Autodesk Inventor part; units mm, degrees
ref_plane "YZ Plane" through (0, 0, 0) normal (1, 0, 0) x (0, 1, 0)
ref_plane "XZ Plane" through (0, 0, 0) normal (0, 1, 0) x (-1, 0, 0)
ref_plane "XY Plane" through (0, 0, 0) normal (0, 0, 1) x (1, 0, 0)
sketch "Sketch1" plane through (0, 0, 0) normal (0, 1, 0) x (-1, 0, 0)
  line L0 (46, 0) -> (-35, 0) construction
  line L1 (0, 54) -> (0, -60) construction
  line L2 (10, 20) -> (-10, 20)
  line L3 (-10, 20) -> (-10, -20)
  line L4 (-10, -20) -> (10, -20)
  line L5 (10, -20) -> (10, 20)
  line L6 (17, -28) -> (17, 28)
  line L7 (17, 28) -> (-13, 28)
  line L8 (-13, 28) -> (-13, -9.5)
  line L9 (-13, -9.5) -> (-36.5, -9.5)
  line L10 (-36.5, -9.5) -> (-36.5, -28)
  line L11 (-36.5, -28) -> (17, -28)
  line L12 (-29.5, -20) -> (-29.5, -17.5)
  line L13 (-10.5, -17.5) -> (-10.5, -20)
  circle A0 centre (5, 24.25) radius 0.5
  circle A1 centre (-5, 24.25) radius 0.5
  line L14 (14.6784, 24.25) -> (-18, 24.25) construction
  circle A2 centre (5, -24.25) radius 0.5
  circle A3 centre (-5, -24.25) radius 0.5
  circle A4 centre (13.5, -18.75) radius 1.5
  circle A5 centre (13.5, 18.75) radius 1.5
  circle A6 centre (-33, -18.75) radius 1.5
  line L15 (-20, 4) -> (-20, -26.5) construction
  line L16 (-10.5, -20) -> (-19.5, -20)
  line L17 (-19.5, -20) -> (-19.5, -22)
  line L18 (-19.5, -22) -> (-20.5, -22)
  line L19 (-20.5, -22) -> (-20.5, -20)
  line L20 (-20.5, -20) -> (-29.5, -20)
  line L21 (-10.5, -17.5) -> (-29.5, -17.5)
  point P0 (0, 0)
  point P1 (-20.5, -17.5)
  dimension "d0" = 40
  dimension "d1" = 20
  dimension "d2" = 7
  dimension "d3" = 8
  dimension "d4" = 8
  dimension "d5" = 3
  dimension "d6" = 20
  dimension "d7" = 10
  dimension "d8" = 19
  dimension "d9" = 2.5
  dimension "d10" = 0.5
  dimension "d11" = 1
  dimension "d12" = 1
  dimension "d13" = 5
  dimension "d14" = 5
  dimension "d15" = 4.25
  dimension "d16" = 3
  dimension "d17" = 9.25
  dimension "d19" = 18.5
  dimension "d20" = 7
  dimension "d21" = 3
  dimension "d23" = 9.25
  dimension "d29" = 3.5
  dimension "d30" = 3.5
  dimension "d31" = 2
  dimension "d32" = 1
extrude "Extrusion1" add sketch "Sketch1" along normal blind 3
fillet "Fillet1" radius 1 6 edges at (-17, 1.5, 28) (13, 1.5, 28) (13, 1.5, -9.5) (36.5, 1.5, -9.5) (36.5, 1.5, -28) (-17, 1.5, -28)
properties part number "BracketCoxa"
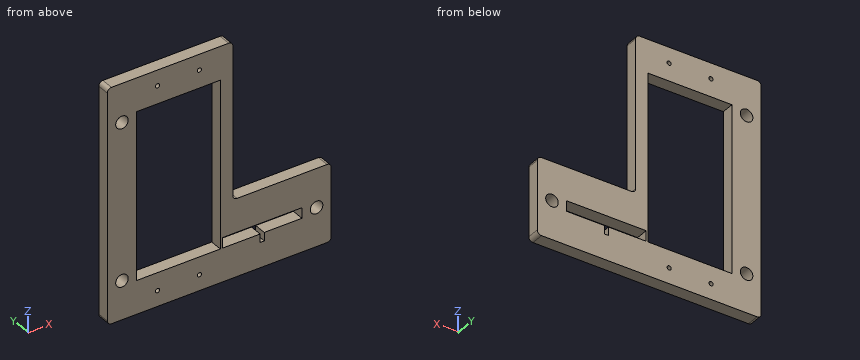
Can you work these out from the model? Positions are in its coordinate system, mm. Coordinates: 2 decimals unless noted, no trailing zeros. Write each loop counter-clockwise with the first axis right and the second up, starting at its lowest first coordinate (ties: lowest second). Pieces come first, ordered by that corner, then holes. Notation, with made-up numbers: (52, 76) - (104, 76) arc R16 cw to (104, 103) - close; hole circle Ø1 at (9.25, 62). An arc over 180 degrees is marked (long way). Return JSON: item names as keys, results as strings. Group by question number.
Item 1: If we section it at A-A (z = 18.75): Write out the boundary of the cut face in (x, y), then the cut area to 3 significant figures.
Item 2: Please list where these lines run through material, in increasing order: probe 1 along Z at (x, y) = (-5, 1.8); probe 2 along Z at (x, y) = (33, 2.1); probe 3 along Z at (x, y) = (12, 0.7).
Item 3: If we section it at D-D (x = -1): Write out the boundary of the cut face in (y, z), then the cut area to 3 significant figures.
Item 4: If we section it at B-B (x = -13.5): Write out the boundary of the cut face in (y, z), then the cut area to 3 significant figures.
Item 5: If we section it at C-C (y = 0.75): Count the separate pieces of the cut face and the enclosed holes in it, then the cut area to 3 significant figures.
Item 6: I'm going to push flat-ended pins straight in: pin 1 Ø0.9 at (x, y) = (14, 1) entering from +Z; pin 2 Ø1.5 at (y, z) = (1.5, -0.5) entering from +X; pin 3 Ø0.9 at (x, y) = (26, 1) entering from +Z. Where does each tip first touch, or does it pass through?
Return value:
{
 "1": {"outline": "(-17, 0) - (-15, 0) - (-15, 3) - (-17, 3) - close; (-12, 0) - (-10, 0) - (-10, 3) - (-12, 3) - close; (10, 0) - (13, 0) - (13, 3) - (10, 3) - close", "area": "21.0 mm^2"},
 "2": {"probe 1": "z = -28 to -24.75, -23.75 to -20, 20 to 23.75, 24.75 to 28", "probe 2": "z = -28 to -20.25, -17.25 to -9.5", "probe 3": "z = -28 to -20, -17.5 to 28"},
 "3": {"outline": "(0, -28) - (3, -28) - (3, -20) - (0, -20) - close; (0, 20) - (3, 20) - (3, 28) - (0, 28) - close", "area": "48.0 mm^2"},
 "4": {"outline": "(0, -28) - (3, -28) - (3, -20.25) - (0, -20.25) - close; (0, -17.25) - (3, -17.25) - (3, 17.25) - (0, 17.25) - close; (0, 20.25) - (3, 20.25) - (3, 28) - (0, 28) - close", "area": "150 mm^2"},
 "5": {"separate pieces": "1", "enclosed holes": "9", "area": "1,240 mm^2"},
 "6": {"pin 1": "stops at z = -9.39", "pin 2": "stops at x = 13", "pin 3": "stops at z = -9.5"}
}
